Build history of the part. All positions in model axes, mm. Face numbers are marked on the shaded views. A direction names the side the tool comes from. Round coordinates to 2 decimals unless told otherwise and drop trailing zeros. Loops run counter-clockwise (first coordinate to the right, second up) from the corner with the lowest first, then second, coordinate; pieces in that order, holes last.
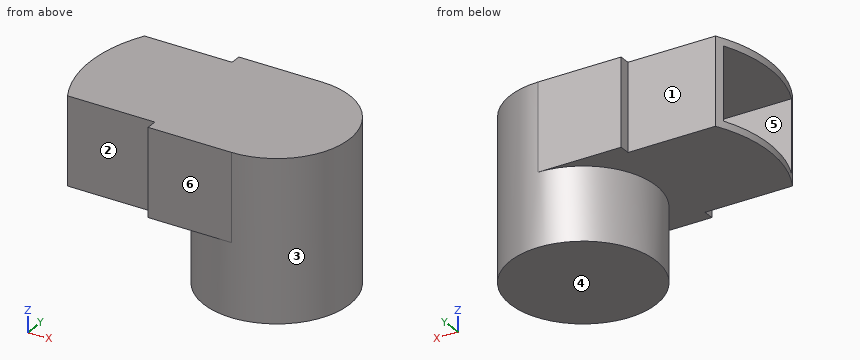
from build123d import *

# Parameters (mm, degrees)
ESQUISSE1_R        = 10
BOSS_EXTRU_1_DEPTH = 10
BOSS_EXTRU_4_DEPTH = 12
COQUE1_START       = 11
COQUE1_DEPTH       = 10
COQUE1_START_2     = 1
COQUE1_2_OUTLINE_R = 9
COQUE1_2_DEPTH     = 10


# Read off the part's stored shape, not the designer's step: Coque1
with BuildPart() as part:
    # Esquisse1 → Boss.-Extru.1 (new body)
    with BuildSketch(Plane.XY):
        Circle(ESQUISSE1_R)
    extrude(amount=BOSS_EXTRU_1_DEPTH)

    # Esquisse5 → Boss.-Extru.4 (add)
    with BuildSketch(Plane.XY.offset(10)):
        with BuildLine():
            Line((-11.427841592, -10), (0, -10))
            ThreePointArc((0, -10), (10, 0), (0, 10))
            Line((0, 10), (-11.427841592, 10))
            Line((-11.427841592, 10), (-11.427841592, 8.5))
            Line((-11.427841592, 8.5), (-23.427841592, 8.5))
            ThreePointArc((-23.427841592, 8.5), (-25.561840174, 0), (-23.427841592, -8.5))
            Line((-23.427841592, -8.5), (-11.427841592, -8.5))
            Line((-11.427841592, -8.5), (-11.427841592, -10))
        make_face()
    extrude(amount=BOSS_EXTRU_4_DEPTH)

    # Coque1 outline → Coque1 (cut)
    with BuildSketch(Plane.XY.offset(COQUE1_START)):
        with BuildLine():
            ThreePointArc((0, -9), (9, 0), (0, 9))
            Line((0, 9), (-10.427841592, 9))
            Line((-10.427841592, 9), (-10.427841592, 7.5))
            Line((-10.427841592, 7.5), (-23.924439446, 7.5))
            ThreePointArc((-23.924439446, 7.5), (-25.561840174, 0), (-23.924439446, -7.5))
            Line((-23.924439446, -7.5), (-10.427841592, -7.5))
            Line((-10.427841592, -7.5), (-10.427841592, -9))
            Line((-10.427841592, -9), (0, -9))
        make_face()
    extrude(amount=COQUE1_DEPTH, mode=Mode.SUBTRACT)

    # Coque1 2 outline → Coque1 2 (cut)
    with BuildSketch(Plane.XY.offset(COQUE1_START_2)):
        Circle(COQUE1_2_OUTLINE_R)
    extrude(amount=COQUE1_2_DEPTH, mode=Mode.SUBTRACT)


solid = part.part
(1) Which spindle directions (+Z, -Z, +X, -X, +Y, -Y) get a long thin tool onto all of the face, cutting with end or side? Do the marked faces 1, 2 and 3. Say none if no direction does.
Responses:
face 1: +Z, -Z, -X, +Y
face 2: +Z, -Z, -X, -Y
face 3: -Z
(2) Slice it at C-C on z = 17.5. List the corners of the cut face in (x, y), plus the area to 3 significant figures.
Responses:
outline: (-23.92, -7.5) arc R18 ccw to (-23.43, -8.5) - (-11.43, -8.5) - (-11.43, -10) - (0, -10) arc R10 ccw to (0, 10) - (-11.43, 10) - (-11.43, 8.5) - (-23.43, 8.5) arc R18 ccw to (-23.92, 7.5) - (-10.43, 7.5) - (-10.43, 9) - (0, 9) arc R9 cw to (0, -9) - (-10.43, -9) - (-10.43, -7.5) - close
area: 80.2 mm2
(3) Slice it at A-A on x = -12.5. List the corners of the cut face in (y, z).
Responses:
outline: (-8.5, 10) - (8.5, 10) - (8.5, 22) - (-8.5, 22) - close; hole (-7.5, 11) - (7.5, 11) - (7.5, 21) - (-7.5, 21) - close
(4) Pin check, flat tips, straight feed: P1, Ø1.2, axis at y = -9, z = 17.5, coming from the -X side; P2, Ø8, axis at x = -17, z = 17, coming from the -Y side; P3, Ø10, axis at x = 6, y = -6.5, coming from the -Z side; P4, Ø1, axis at y = 0, z = 12.5, coming from the -X side. Stop position of each tip, or through.
Responses:
P1: stops at x = -23.48
P2: stops at y = -8.5
P3: stops at z = 0
P4: stops at x = 8.99
(5) Pull direction Y, two halves, no side cores. Call the marked faces 4, 5 and 6: +Y half, -Y half, draft (parallel to the pull), parting line (faces both ways), or undercut.
Responses:
face 4: draft
face 5: undercut
face 6: -Y half
(6) Slice it at B-B on y = 0. List the corners of the cut face in (x, z).
Responses:
outline: (-25.56, 10) - (-10, 10) - (-10, 0) - (10, 0) - (10, 22) - (-25.56, 22) - (-25.56, 21) - (9, 21) - (9, 1) - (-9, 1) - (-9, 11) - (-25.56, 11) - close
(7) Slice it at D-D on z = 8.5. List the corners of the cut face in (x, y).
Responses:
outline: circle Ø20 at (0, 0); hole circle Ø18 at (0, 0)
(8) Probe line 1 (X direction, y = 0.25, z = 2.5); line 2 (Z direction, x = -0.5, y = -3); line 3 (Z direction, x = -20.5, y = -1.5). List the from-to ranges inside material, lowest first.
Responses:
line 1: x = -10 to -9, 9 to 10
line 2: z = 0 to 1, 21 to 22
line 3: z = 10 to 11, 21 to 22
